Source: CAD feature listing. Evaluate the final solid. Frame: model axes, mm. A direction names the side the tool comes from. Give positions to 0.01 mm unless a question says otherwise; leave off trailing zeros. Order: outer loops, then holes, each group sorted by start corner. A loop starts at its lowest first (then second) coordinate and runs counter-clockwise, first axis right, second up. Notation, with made-up numbers: M 59,-34.75 L 65,-34.75 A20 cw 65,-8.75 Z; hole C 31.25,27 d11. An arc over 180 degrees is marked long. Return JSON: item names as keys, results as strings.
from build123d import *

# Parameters (mm, degrees)
SKETCH_1_R      = 1.5
EXTRUDE_1_DEPTH = 47
SKETCH_2_R      = 11
EXTRUDE_2_DEPTH = 2
SKETCH_3_R      = 2.5
EXTRUDE_3_DEPTH = 20
SKETCH_4_W      = 16
SKETCH_4_H      = 6
EXTRUDE_4_DEPTH = 6


with BuildPart() as part:
    # 草图1 → 凸台-拉伸1 (new body)
    with BuildSketch(Plane.XY):
        Polygon((21, 0), (21, 16.6), (16.6, 21), (0, 21), (-16.6, 21), (-21, 16.6), (-21, 0), (-21, -16.6), (-16.6, -21), (0, -21), (16.6, -21), (21, -16.6), align=None)
        with Locations((15.5, 15.5)):
            Circle(SKETCH_1_R, mode=Mode.SUBTRACT)
        with Locations((15.5, -15.5)):
            Circle(SKETCH_1_R, mode=Mode.SUBTRACT)
        with Locations((-15.5, -15.5)):
            Circle(SKETCH_1_R, mode=Mode.SUBTRACT)
        with Locations((-15.5, 15.5)):
            Circle(SKETCH_1_R, mode=Mode.SUBTRACT)
    extrude(amount=EXTRUDE_1_DEPTH)

    # 草图2 → 凸台-拉伸2 (add)
    with BuildSketch(Plane.XY.offset(47)):
        Circle(SKETCH_2_R)
    extrude(amount=EXTRUDE_2_DEPTH)

    # 草图3 → 凸台-拉伸3 (add)
    with BuildSketch(Plane.XY.offset(47)):
        Circle(SKETCH_3_R)
    extrude(amount=EXTRUDE_3_DEPTH)

    # 草图4 → 凸台-拉伸4 (add)
    with BuildSketch(Plane(origin=(0, 21, 0), x_dir=(1, 0, 0), z_dir=(0, 1, 0))):
        with Locations((0, -6)):
            Rectangle(SKETCH_4_W, SKETCH_4_H)
    extrude(amount=EXTRUDE_4_DEPTH)


solid = part.part
1. Set-up query: faces 5 (the face through (0, 24, 3)), 6 (the face through (-8, 24, 6)), 7 (the face through (-18.8, -18.8, 23.2)), 8 (the face through (-2.38, -10.74, 47.99)), 9 (the face through (0, 27, 6)). Return all of +Z, -Z, +X, -X, +Y, -Y with unobstructed straight access to the full face (end or side cutting, diameter ignored); none if empty.
Evaluation:
{"face 5": "-Z, +X, -X, +Y", "face 6": "+Z, -Z, -X, +Y", "face 7": "+Z, -Z, -X, -Y", "face 8": "+Z", "face 9": "+Z, -Z, +X, -X, +Y"}
2. First-contact query: pin 1 (2.5 mm diameter, centred on x = -15.5, y = 15.5, fed in from +Z); pin 2 (1 mm diameter, centred on x = 5, z = 30.5, fed in from +Y); pin 3 (3 mm diameter, centred on x = 6, y = -4, fed in from +Z); pin 4 (5 mm diameter, centred on x = -1.5, y = 25, fed in from +Z). Flat tips, straight axial feed; report the tip coordinate or a pass-through.
Evaluation:
{"pin 1": "passes through", "pin 2": "stops at y = 21", "pin 3": "stops at z = 49", "pin 4": "stops at z = 9"}
3. Section query D-D (y = 0). Return loops of the section in (x, z), then the cut area to 3 significant figures.
Evaluation:
{"outline": "M -21,0 L 21,0 L 21,47 L 11,47 L 11,49 L 2.5,49 L 2.5,67 L -2.5,67 L -2.5,49 L -11,49 L -11,47 L -21,47 Z", "area": "2,110 mm^2"}
4. Draft query along Y for faces 1 (the face through (14, -15.43, 23.17)), 2 (the face through (-18.8, 18.8, 23.2)), 3 (the face through (8, 24, 6)), 4 (the face through (-17, 15.57, 23.17)). Return one class per face: pulls with the +Y half, pulls with the -Y half, needs draft (parallel to the pull), parting line crosses it, or undercut.
Evaluation:
{"face 1": "undercut", "face 2": "pulls with the +Y half", "face 3": "needs draft", "face 4": "undercut"}
5. Section query A-A (y = -15.5). Return loops of the section in (x, z), then the cut area to 3 significant figures.
Evaluation:
{"outline": "M -21,0 L -17,0 L -17,47 L -21,47 Z; M -14,0 L 14,0 L 14,47 L -14,47 Z; M 17,0 L 21,0 L 21,47 L 17,47 Z", "area": "1,690 mm^2"}
6. Section query B-B (z = 30). Return loops of the section in (x, y), then the cut area to 3 significant figures.
Evaluation:
{"outline": "M -21,-16.6 L -16.6,-21 L 16.6,-21 L 21,-16.6 L 21,16.6 L 16.6,21 L -16.6,21 L -21,16.6 Z; hole C -15.5,-15.5 d3; hole C -15.5,15.5 d3; hole C 15.5,-15.5 d3; hole C 15.5,15.5 d3", "area": "1,700 mm^2"}
7. Ray query, probe 1 along Y at (x, z) = (15.5, 17); probe 2 along Y at (x, z) = (-15, 13); probe 3 along Z at (x, y) = (-18, 10.5). Return the intervals inside material, ascending.
Evaluation:
{"probe 1": "y = -21 to -17, -14 to 14, 17 to 21", "probe 2": "y = -21 to -16.91, -14.09 to 14.09, 16.91 to 21", "probe 3": "z = 0 to 47"}
